Geometry: see drawing. Coordinates: mm, zero at the bounding-box minimum. Coordinates: 2 decimals unless noted, no trailing zeros. Write each loop counter-clockwise with the first axis right and the second up, starting at its lowest first coordinate (ties: lowest second). Pieces come first, ordered by that corner, then holes.
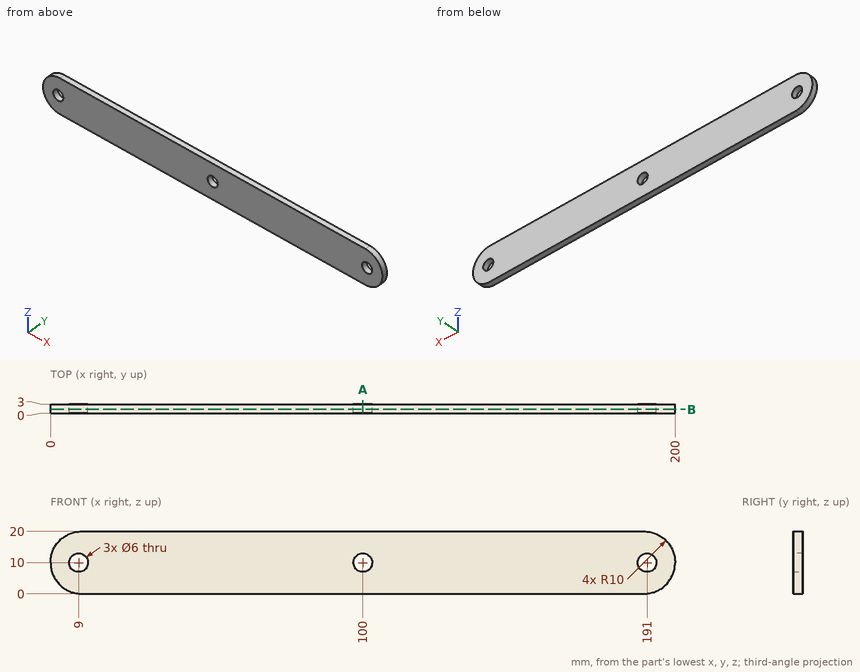
Item 1: Pin query (flat end, axial travel): pin 1 (5 mm diameter, centred on x = 191, z = 10, fed in from -Y). Return the tip coordinate at first contact, or that it passes through.
Derived:
pin 1: passes through
Item 2: Material intervals for probe 1 along X at (y, z) = (0.8, 10); probe 2 along X at (y, z) = (1.35, 8.25); probe 3 along Z at (x, y) = (191, 1.2), sorted ascending.
Derived:
probe 1: x = 0 to 6, 12 to 97, 103 to 188, 194 to 200
probe 2: x = 0.15 to 6.56, 11.44 to 97.56, 102.44 to 188.56, 193.44 to 199.85
probe 3: z = 0.05 to 7, 13 to 19.95
Item 3: Section B-B, the plane y = 1.3. State how many separate pieces and enclosed holes the cut face has, plus the area to 3 significant figures.
Derived:
separate pieces: 1
enclosed holes: 3
area: 3,830 mm2
Item 4: Section A-A, the plane x = 100. Output: boundary loops of the cut face in (y, z), plus the area to 3 significant figures.
Derived:
outline: (0, 0) - (3, 0) - (3, 7) - (0, 7) - close; (0, 13) - (3, 13) - (3, 20) - (0, 20) - close
area: 42.0 mm2
